from build123d import *

# Parameters (mm, degrees)
FORMSENKUNG_F_R_M3_SENKSCHRAUBE_MIT_INNE_D           = 3.4
FORMSENKUNG_F_R_M3_SENKSCHRAUBE_MIT_INNE_CSINK_D     = 5.7
FORMSENKUNG_F_R_M3_SENKSCHRAUBE_MIT_INNE_CSINK_ANGLE = 90
KREISMUSTER1_COUNT                                   = 4
SKIZZE5_R                                            = 24.563351151
SKIZZE5_R_2                                          = 12.292484408
SCHNITT_LINEAR_AUSTRAGEN3_DEPTH                      = 32.128764833
SCHNITT_LINEAR_AUSTRAGEN5_DEPTH                      = 29.565713714
SCHNITT_LINEAR_AUSTRAGEN5_DEPTH_BACK                 = 29.565713714
SKIZZE12_R                                           = 25.145284477
SKIZZE12_R_2                                         = 13.9
SCHNITT_LINEAR_AUSTRAGEN6_DEPTH                      = 21.06040877
SCHNITT_LINEAR_AUSTRAGEN6_DEPTH_BACK                 = 21.06040877
SKIZZE13_R                                           = 6.1


with BuildPart() as part:
    # Skizze1 → Rotation1 (revolve)
    with BuildSketch(Plane.XY, mode=Mode.PRIVATE) as rotation1_sk:
        Polygon((-30.239658347, 20), (-30.239658347, 6), (-26.239658347, 6), (-26.239658347, 10), (-27.239658347, 10), (-27.239658347, 14), (-14.239658347, 14), (-14.239658347, 20), align=None)
    revolve(rotation1_sk.sketch.rotate(Axis((-37.668433178, 0, 0), (1, 0, 0)), 90), axis=Axis((-37.668433178, 0, 0), (1, 0, 0)))

    # Formsenkung f_r M3 Senkschraube mit Inne (through all)
    with Locations(Plane(origin=(-14.239658347, 0, 0), x_dir=(0, 0, -1), z_dir=(1, 0, 0))):
        with Locations((0, 17)):
            formsenkung_f_r_m3_senkschraube_mit_inne = CounterSinkHole(FORMSENKUNG_F_R_M3_SENKSCHRAUBE_MIT_INNE_D / 2, FORMSENKUNG_F_R_M3_SENKSCHRAUBE_MIT_INNE_CSINK_D / 2, counter_sink_angle=FORMSENKUNG_F_R_M3_SENKSCHRAUBE_MIT_INNE_CSINK_ANGLE)

    # Kreismuster1: Formsenkung f_r M3 Senkschraube mit Inne ×4 about axis
    kreismuster1_axis = Axis((0, 0, 0), (1, 0, 0))
    for i in range(1, KREISMUSTER1_COUNT):
        add(formsenkung_f_r_m3_senkschraube_mit_inne.rotate(kreismuster1_axis, i * 360 / KREISMUSTER1_COUNT), mode=Mode.SUBTRACT)

    # Skizze5 → Schnitt-Linear austragen3 (cut, through all)
    with BuildSketch(Plane(origin=(-27.239658347, 0, 0), x_dir=(0, 0, -1), z_dir=(1, 0, 0))):
        Circle(SKIZZE5_R)
        Circle(SKIZZE5_R_2, mode=Mode.SUBTRACT)
    extrude(amount=SCHNITT_LINEAR_AUSTRAGEN3_DEPTH, mode=Mode.SUBTRACT)

    # Skizze12 → Schnitt-Linear austragen5 (cut, two sides: drawn at the far end of the back side and taken through both)
    with BuildSketch(Plane(origin=(-26.239658347, 0, 0), x_dir=(0, 0, -1), z_dir=(1, 0, 0)).offset(-SCHNITT_LINEAR_AUSTRAGEN5_DEPTH_BACK)):
        Circle(SKIZZE12_R)
        Circle(SKIZZE12_R_2, mode=Mode.SUBTRACT)
    extrude(amount=SCHNITT_LINEAR_AUSTRAGEN5_DEPTH + SCHNITT_LINEAR_AUSTRAGEN5_DEPTH_BACK, mode=Mode.SUBTRACT)

    # Skizze13 → Schnitt-Linear austragen6 (cut, two sides: drawn at the far end of the back side and taken through both)
    with BuildSketch(Plane(origin=(-26.239658347, 0, 0), x_dir=(0, 0, -1), z_dir=(1, 0, 0)).offset(-SCHNITT_LINEAR_AUSTRAGEN6_DEPTH_BACK)):
        Circle(SKIZZE13_R)
    extrude(amount=SCHNITT_LINEAR_AUSTRAGEN6_DEPTH + SCHNITT_LINEAR_AUSTRAGEN6_DEPTH_BACK, mode=Mode.SUBTRACT)


solid = part.part
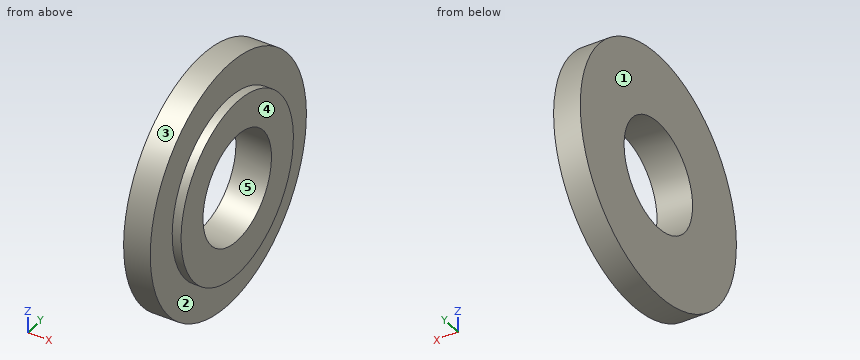
For this review, take the finished solid that the model builds, in its own axes (mm). Face numbers are marked on the shaded views. A direction names the side the tool comes from. Coordinates: 2 decimals unless noted, no trailing zeros. Loops run counter-clockwise (first coordinate to the right, second up) from the corner with the lowest first, then second, coordinate; pieces in that order, holes last. Notation, with made-up numbers: (42.25, 56) - (72.25, 56) arc R17 cw to (72.25, 68) - close; hole circle Ø2 at (47.25, -19.5). An arc over 180 degrees is marked (long way). Use a Markdown table: item, result. Add a question column.
Item 1: For line 1 (Y direction, x = -28.8, z = 0); line 2 (Y direction, x = -26.95, z = 0), list the stretches that pass through material, from the lowest coordinate up.
Item 2: We need section D-D (z = -6.5). Give the boundary of the cut face in (x, y), and give its area (3 significant figures).
Item 3: We need section A-A (y = 0). Give the boundary of the cut face in (x, z), and give its area (3 significant figures).
Item 4: We need section C-C (x = -28.6). Give the boundary of the cut face in (y, z).
Item 5: We need section B-B (z = 3). Give the boundary of the cut face in (x, y).
Item 6: Mouldability with a two-part tool opening along Y and no side actions: class the marked faces 3, 4 and 5 as pulls with the +Y half, pulls with the -Y half, needs draft (parallel to the pull), parting line crosses it, or undercut.
Item 7: Tool access review of the marked faces 1 and 2: name each direction out of +Z, -Z, +X, -X, +Y, -Y from which nothing blocks a thin tool from reaching the whole face with its end or side.
Item 8: Insertion check: pin 1 Ø2 at (x, z) = (-29, -10.5) entering from -Y; pin 2 Ø1.5 at (x, y) = (-30, -3) entering from -Z; pin 3 Ø1 at (x, z) = (-29.5, -11) entering from -Y. Each pin has a flat end and moves straight along its axis. Give the tip position at first contact, or say it passes through.
Results list:
| question | item | result |
|---|---|---|
| 1 | line 1 | y = -13.9 to -6.1, 6.1 to 13.9 |
| 1 | line 2 | y = -10 to -6.1, 6.1 to 10 |
| 2 | outline | (-30.24, -12.29) - (-27.24, -12.29) - (-27.24, -7.6) - (-26.24, -7.6) - (-26.24, 7.6) - (-27.24, 7.6) - (-27.24, 12.29) - (-30.24, 12.29) - close |
| 2 | area | 88.9 mm^2 |
| 3 | outline | (-30.24, -13.9) - (-27.24, -13.9) - (-27.24, -10) - (-26.24, -10) - (-26.24, -6.1) - (-30.24, -6.1) - close; (-30.24, 6.1) - (-26.24, 6.1) - (-26.24, 10) - (-27.24, 10) - (-27.24, 13.9) - (-30.24, 13.9) - close |
| 3 | area | 54.6 mm^2 |
| 4 | outline | circle Ø27.8 at (0, 0); hole circle Ø12.2 at (0, 0) |
| 5 | outline | (-30.24, -13.57) - (-27.24, -13.57) - (-27.24, -9.54) - (-26.24, -9.54) - (-26.24, -5.31) - (-30.24, -5.31) - close; (-30.24, 5.31) - (-26.24, 5.31) - (-26.24, 9.54) - (-27.24, 9.54) - (-27.24, 13.57) - (-30.24, 13.57) - close |
| 6 | face 3 | parting line crosses it |
| 6 | face 4 | needs draft |
| 6 | face 5 | undercut |
| 7 | face 1 | +Z, -Z, -X, +Y, -Y |
| 7 | face 2 | +X |
| 8 | pin 1 | stops at y = -10.15 |
| 8 | pin 2 | stops at z = -13.72 |
| 8 | pin 3 | stops at y = -9.11 |
